Autodesk Inventor part; units mm, degrees
ref_plane "YZ Plane" through (0, 0, 0) normal (1, 0, 0) x (0, 1, 0)
ref_plane "XZ Plane" through (0, 0, 0) normal (0, 1, 0) x (-1, 0, 0)
ref_plane "XY Plane" through (0, 0, 0) normal (0, 0, 1) x (1, 0, 0)
sketch "Sketch1" plane through (0, 0, 0) normal (0, 0, 1) x (1, 0, 0)
  line L0 (0, -6) -> (0, -3) construction
  line L1 (2.25, -3.75) -> (0, -6) construction
  line L2 (2.25, -3.75) -> (0, -6)
  line L3 (0, -6) -> (0, -3)
  line L4 (0, -3) -> (0, 0)
  line L5 (0.75, -2.25) -> (3, 0) construction
  line L6 (2.25, -3.75) -> (0.75, -2.25)
  line L7 (3, 0) -> (0.75, -2.25)
  line L8 (0, 0) -> (3, 0)
  point P0 (0, -1.5)
extrude "Extrusion1" add sketch "Sketch1" along normal blind 63
sketch "Sketch2" plane through (0, 0, 0) normal (0, 1, 0) x (1, 0, 0)
  line L0 (0.75, -63) -> (3, -63)
  line L1 (3, -63) -> (-2, -63)
  line L2 (-2, -63) -> (-2, 0)
  line L3 (-2, 0) -> (3, 0)
  line L4 (3, 0) -> (3, -63)
  point P0 (0, 0)
  dimension "d2" = 5
  dimension "d3" = 63
extrude "Extrusion2" add sketch "Sketch2" along normal blind 0.5
sketch "Sketch3" plane through (0, 0.5, 0) normal (0, 1, 0) x (1, 0, 0)
  line L0 (0.75, -63) -> (3, -63)
  line L1 (3, -63) -> (-5, -63)
  line L2 (-5, -63) -> (-5, 0)
  line L3 (-5, 0) -> (3, 0)
  line L4 (3, 0) -> (3, -63)
  point P0 (0, 0)
  dimension "d6" = 63
  dimension "d7" = 8
extrude "Extrusion3" add sketch "Sketch3" along normal blind 3
properties part number "SlidingLock"
Verification items for the finished model (mm, model axes). A direction names the side the tool comes from. Give positions to 0.01 mm unless a question says otherwise; leave off trailing zeros. Loops run counter-clockwise (first coordinate to the right, second up) from the corner with the lowest first, then second, coordinate; pieces in that order, holes last. Notation, with made-up numbers: M 18.5,3.5 L 64.5,3.5 A24 ccw 64.5,20.5 Z; hole C -19,89 d2. An arc over 180 degrees is marked long. Return JSON: item names as keys, results as strings.
1) Gauge pin test, flat ends, axial feed: P1, Ø0.6, axis at x = -1.5, z = 17, coming from the -Y side; P2, Ø3.5, axis at x = -4, z = 28, coming from the -Y side. Record the tip position at first contact, or that the pin passes through.
Findings:
{"P1": "stops at y = 0", "P2": "stops at y = 0.5"}
2) Section check B-B, the plane y = -5. Enter the section's corners in (x, z), and give its area (3 significant figures).
Findings:
{"outline": "M 0,0 L 1,0 L 1,63 L 0,63 Z", "area": "63.0 mm2"}
3) Material ranges on L1, parallel to Y at x = -3.25, z = 30; L2, parallel to Y at x = 2, z = 59; L3, parallel to X at y = -3, z = 14, recorded low to high. Write a range as [from, to].
Findings:
{"L1": "y = [0.5, 3.5]", "L2": "y = [-4, -3.5], [-1, 3.5]", "L3": "x = [0, 1.5]"}
4) Section check A-A, the plane z = 28.5. Enter the section's corners in (x, y).
Findings:
{"outline": "M -5,0.5 L -2,0.5 L -2,0 L 0,0 L 0,-6 L 2.25,-3.75 L 0.75,-2.25 L 3,0 L 3,3.5 L -5,3.5 Z"}
5) Tool access check on faces 1 (the flat face through (0, 1, 63)), 2 (the flat face through (-4, 0.5, 31)), 3 (the flat face through (2, -1, 31)). Record the directions out of +Z, -Z, +X, -X, +Y, -Y that give a thin tool (end or side, any length) a straight path to the whole face; none if there is none.
Findings:
{"face 1": "+Z, +X, -X, +Y, -Y", "face 2": "+Z, -Z, -X, -Y", "face 3": "+Z, -Z, +X"}
6) Mould release check, pull along Y, two halves, no side actions. Record for faces 4 (the flat face through (0, -3, 31)), 5 (the flat face through (-1, 3.5, 31)), 6 (the flat face through (1.5, -3, 31.1)): released by +Y, released by -Y, zero draft, split by the parting line, or undercut.
Findings:
{"face 4": "zero draft", "face 5": "released by +Y", "face 6": "undercut"}
7) Section check C-C, the plane x = -3.25. Enter the section's corners in (y, z).
Findings:
{"outline": "M 0.5,0 L 3.5,0 L 3.5,63 L 0.5,63 Z"}
